Source: three-view drawing plus pictorial views. Frame: mm from the lowest corner of the part. Give positions to 0.01 mm unless a question says otherwise; leave off trailing zeros. Order: outer loops, then holes, each group sorted by start corner. A loop starts at its lowest first (then second) coordinate and runs counter-clockwise, first axis right, second up. Notation, with made-up numbers: (-0.75, -34.75) - (54.25, -34.75) arc R14 ccw to (54.25, -24.75) - close; hole circle Ø9 at (74, -0.5). An arc over 180 degrees is marked (long way). Answer in a Markdown table with one row per item. Add a question column.
1. Contact query for a flat-ended pin moving along its axis: pin 1 (1.8 mm diameter, centred on x = 7, z = 47, fed in from +Y). Output: stop coordinate, or through.
2. Ray query, line 1 (X direction, y = 4.75, z = 88.5); line 2 (Y direction, x = 2.5, z = 62). Return the intervals inside material, ascending. Write a range as [from, to].
3. Section query A-A on y = 6.5. Return loops of the section in (x, z).
4. Section query C-C on x = 2.75. Return loops of the section in (y, z), and give its area (3 significant figures).
5. Section query B-B on z = 41. Return loops of the section in (x, y), and give its area (3 significant figures).
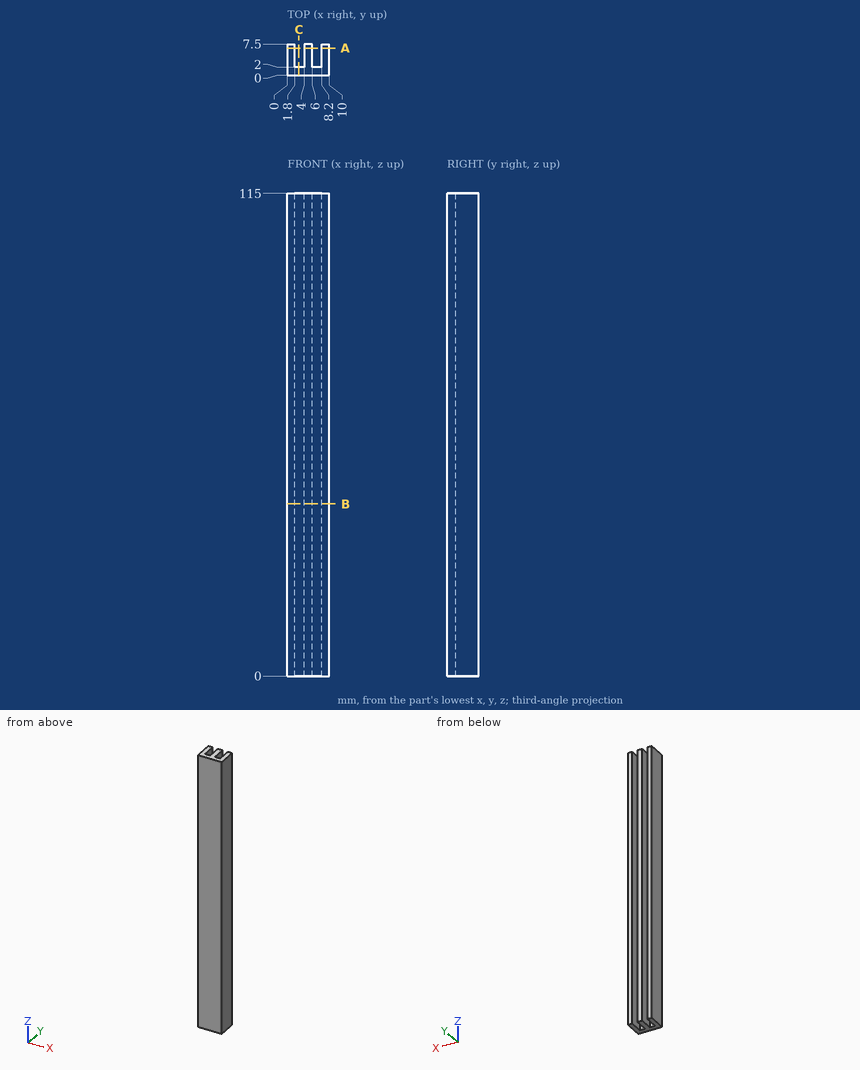
Answer:
| question | item | result |
|---|---|---|
| 1 | pin 1 | stops at y = 2 |
| 2 | line 1 | x = [0, 1.8], [4, 6], [8.2, 10] |
| 2 | line 2 | y = [0, 2] |
| 3 | outline | (0, 0) - (1.8, 0) - (1.8, 115) - (0, 115) - close; (4, 0) - (6, 0) - (6, 115) - (4, 115) - close; (8.2, 0) - (10, 0) - (10, 115) - (8.2, 115) - close |
| 4 | outline | (0, 0) - (2, 0) - (2, 115) - (0, 115) - close |
| 4 | area | 230 mm² |
| 5 | outline | (0, 0) - (10, 0) - (10, 7.5) - (8.2, 7.5) - (8.2, 2) - (6, 2) - (6, 7.5) - (4, 7.5) - (4, 2) - (1.8, 2) - (1.8, 7.5) - (0, 7.5) - close |
| 5 | area | 50.8 mm² |
